Design review of the part shown in the three views and the two pictorial views. Dimensions are in mm from the part's minimum x, y and z. A direction names the side the tool comes from. Coordinates: 2 decimals unless noted, no trailing zeros. Loops run counter-clockwise (first coordinate to the right, second up) from the corner with the lowest first, then second, coordinate; pieces in that order, holes last. Notation, with made-up numbers: (16, 85) -> (25, 85) arc R19 ccw to (25, 119) -> close; hole circle Ø8 at (64.25, 46). An arc over 180 degrees is marked (long way). Answer in a Markdown table with one row per item.
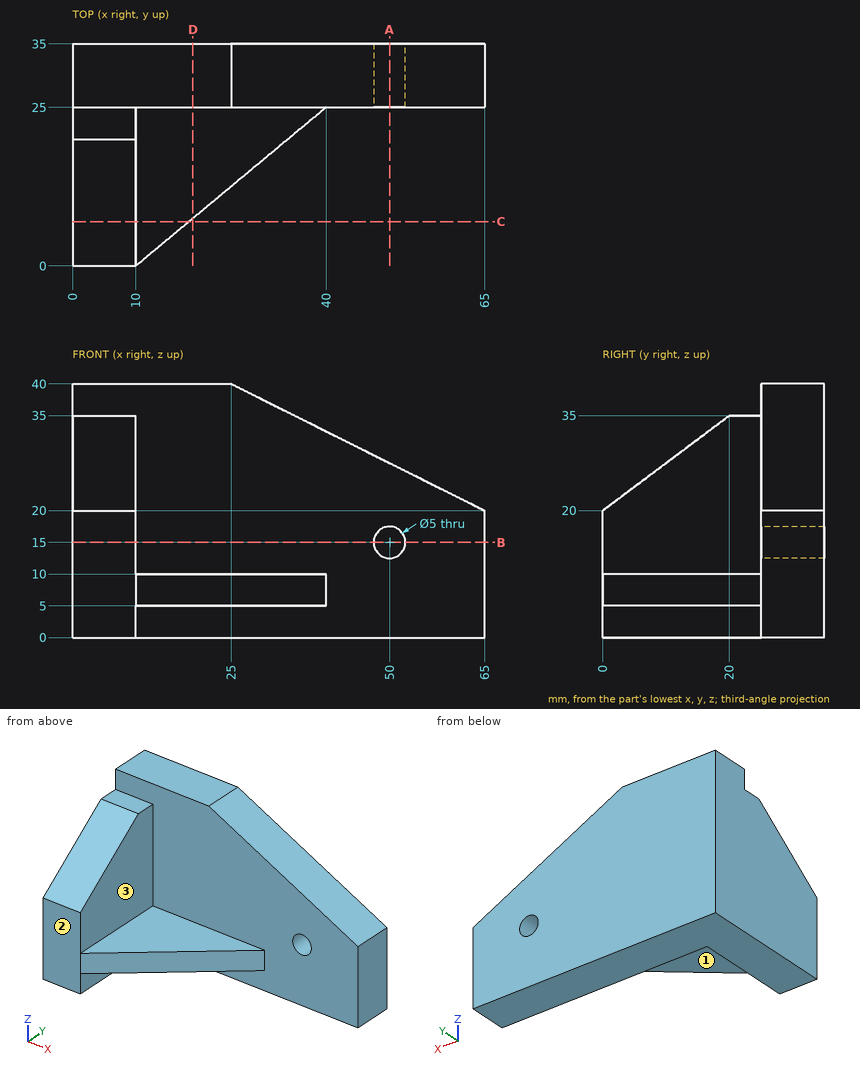
Item 1: Take a section at C-C, the plane y = 7. State the section outline as (x, z) points, and give its area (4 significant figures).
Worked answers:
| item | result |
|---|---|
| outline | (0, 0) -> (10, 0) -> (10, 5) -> (18.4, 5) -> (18.4, 10) -> (10, 10) -> (10, 25.25) -> (0, 25.25) -> close |
| area | 294.5 mm² |
Item 2: Take a section at B-B, the plane z = 15. State the section outline as (x, y) points.
Worked answers:
| item | result |
|---|---|
| outline | (0, 0) -> (10, 0) -> (10, 25) -> (47.5, 25) -> (47.5, 35) -> (0, 35) -> close; (52.5, 25) -> (65, 25) -> (65, 35) -> (52.5, 35) -> close |
Item 3: Take a section at D-D, the plane x = 19. State the section outline as (y, z) points, and give its area (4 significant figures).
Worked answers:
| item | result |
|---|---|
| outline | (7.5, 5) -> (25, 5) -> (25, 0) -> (35, 0) -> (35, 40) -> (25, 40) -> (25, 10) -> (7.5, 10) -> close |
| area | 487.5 mm² |
Item 4: For the marked faces 1, 2 and 3, list the 3-axis set-ups (+Z, -Z, +X, -X, +Y, -Y) from which the entire face can be reached by the end or side of a thin tool; tool diameter is ignored.
Worked answers:
| item | result |
|---|---|
| face 1 | -Z, +X, -Y |
| face 2 | +Z, -Z, +X, -X, -Y |
| face 3 | +Z, +X, -Y |
Item 5: Insertion check: pin 1 (12.5 mm diameter, centred on x = 23.5, y = 8.5, fed in from +Z); pin 2 (4 mm diameter, centred on x = 38, y = 23.5, fed in from +Z); pin 3 (1.5 mm diameter, centred on x = 5.5, y = 21.5, fed in from +Z). Each pin has a flat end and moves straight along its axis. Give the tip position at first contact, or say it passes through.
Worked answers:
| item | result |
|---|---|
| pin 1 | z = 10 |
| pin 2 | z = 34.16 |
| pin 3 | z = 35 |
Item 6: Take a section at A-A, the plane x = 50. State the section outline as (y, z) points.
Worked answers:
| item | result |
|---|---|
| outline | (25, 0) -> (35, 0) -> (35, 12.5) -> (25, 12.5) -> close; (25, 17.5) -> (35, 17.5) -> (35, 27.5) -> (25, 27.5) -> close |
Item 7: For L1, parallel to Y at x = 23.5, z = 4; L2, parallel to Z at x = 50, y = 32.75; L3, parallel to X at y = 21, z = 11, list the stretches that pass through material, from the lowest coordinate up.
Worked answers:
| item | result |
|---|---|
| L1 | 25 to 35 |
| L2 | 0 to 12.5, 17.5 to 27.5 |
| L3 | 0 to 10 |
